Geometry check sheet. Reference: the model listing, model coordinates, mm. A direction names the side the tool comes from. Give positions to 0.01 mm unless a question says otherwise; leave off trailing zeros. Loops run counter-clockwise (first coordinate to the right, second up) from the corner with the lowest first, then second, coordinate; pieces in that order, holes last. Notation, with made-up numbers: (-33.5, 89) -> (23.5, 89) arc R29 cw to (23.5, 110) -> close; hole circle Ø2 at (4.25, -2). An arc over 180 degrees is marked (long way). One line per question, with ' | ' between items.
from build123d import *

# Parameters (mm, degrees)
SKETCH1_W                = 18
SKETCH1_H                = 40
BOSS_EXTRUDE1_DEPTH      = 6
BOSS_EXTRUDE2_DEPTH      = 14
SKETCH3_R                = 4.125
CUT_EXTRUDE1_DEPTH       = 30.681644159
FILLET1_R                = 7
SKETCH12_W               = 3
SKETCH12_H               = 8.5
CUT_EXTRUDE7_DEPTH       = 11.875
SKETCH13_R               = 1.5
CUT_EXTRUDE8_DEPTH       = 25.940241077
CUT_EXTRUDE9_REACH       = 32.725
SKETCH14_R               = 3
CUT_EXTRUDE10_REACH      = 35.526
SKETCH15_W               = 7
SKETCH15_H               = 5.5
SKETCH7_W                = 15.875
SKETCH7_H                = 6
BOSS_EXTRUDE3_DEPTH      = 7
FILLET2_R                = 7
SKETCH8_R                = 2.625
CUT_EXTRUDE4_DEPTH       = 30.189039039
BOSS_EXTRUDE4_DEPTH      = 2.5
BOSS_EXTRUDE4_DEPTH_BACK = 2.5
SKETCH10_R               = 4.875
CUT_EXTRUDE5_DEPTH       = 3


with BuildPart() as part:
    # Sketch1 → Boss-Extrude1 (new body)
    with BuildSketch(Plane(origin=(0, 0, 0), x_dir=(1, 0, 0), z_dir=(0, 1, 0))):
        Rectangle(SKETCH1_W, SKETCH1_H)
    extrude(amount=BOSS_EXTRUDE1_DEPTH)

    # Sketch2 → Boss-Extrude2 (add)
    with BuildSketch(Plane(origin=(0, 6, 0), x_dir=(1, 0, 0), z_dir=(0, 1, 0))):
        with BuildLine():
            Line((3, -20), (3, -8))
            ThreePointArc((3, -8), (-1, 0), (3, 8))
            Line((3, 8), (3, 20))
            Line((3, 20), (9, 20))
            Line((9, 20), (9, -20))
            Line((9, -20), (3, -20))
        make_face()
    extrude(amount=BOSS_EXTRUDE2_DEPTH)

    # Sketch3 → Cut-Extrude1 (cut, through all)
    with BuildSketch(Plane(origin=(0, 20, 0), x_dir=(1, 0, 0), z_dir=(0, 1, 0))):
        with Locations((9, 0)):
            Circle(SKETCH3_R)
    extrude(amount=-CUT_EXTRUDE1_DEPTH, mode=Mode.SUBTRACT)

    # Fillet1
    fillet1_edges = [part.edges().sort_by_distance(p)[0] for p in [
        (6, 20, 20),
        (6, 20, -20),
    ]]
    fillet(fillet1_edges, radius=FILLET1_R)

    # Sketch12 → Cut-Extrude7 (cut)
    with BuildSketch(Plane(origin=(0, 20, 0), x_dir=(1, 0, 0), z_dir=(0, 1, 0))):
        with Locations((5.25, 13)):
            Rectangle(SKETCH12_W, SKETCH12_H)
        with Locations((5.25, -13)):
            Rectangle(SKETCH12_W, SKETCH12_H)
    extrude(amount=-CUT_EXTRUDE7_DEPTH, mode=Mode.SUBTRACT)

    # Sketch13 → Cut-Extrude8 (cut, through all)
    with BuildSketch(Plane(origin=(0, 8.125, 0), x_dir=(1, 0, 0), z_dir=(0, 1, 0))):
        with Locations(Location((5.25, 13, 0), (0, 0, 270))):
            Circle(SKETCH13_R)
        with Locations((5.25, -13)):
            Circle(SKETCH13_R)
    extrude(amount=-CUT_EXTRUDE8_DEPTH, mode=Mode.SUBTRACT)

    # Sketch14 → Cut-Extrude9 (cut, up to next)
    with BuildSketch(Plane.ZY.offset(-3), mode=Mode.PRIVATE) as cut_extrude9_sk1:
        with Locations((-13, 13)):
            Circle(SKETCH14_R)
    cut_extrude9_tool1 = extrude(cut_extrude9_sk1.sketch, amount=-CUT_EXTRUDE9_REACH, mode=Mode.PRIVATE) & part.part
    # Sketch14 → Cut-Extrude9 (cut, up to next)
    with BuildSketch(Plane.ZY.offset(-3), mode=Mode.PRIVATE) as cut_extrude9_sk2:
        with Locations((13, 13)):
            Circle(SKETCH14_R)
    cut_extrude9_tool2 = extrude(cut_extrude9_sk2.sketch, amount=-CUT_EXTRUDE9_REACH, mode=Mode.PRIVATE) & part.part
    add(cut_extrude9_tool1.solids().sort_by_distance((3, 13, -13))[0], mode=Mode.SUBTRACT)
    add(cut_extrude9_tool2.solids().sort_by_distance((3, 13, 13))[0], mode=Mode.SUBTRACT)

    # Sketch15 → Cut-Extrude10 (cut, up to next)
    with BuildSketch(Plane(origin=(9, 0, 0), x_dir=(0, 0, -1), z_dir=(1, 0, 0)), mode=Mode.PRIVATE) as cut_extrude10_sk1:
        with Locations((13, 13)):
            Rectangle(SKETCH15_W, SKETCH15_H)
    cut_extrude10_tool1 = extrude(cut_extrude10_sk1.sketch, amount=-CUT_EXTRUDE10_REACH, mode=Mode.PRIVATE) & part.part
    # Sketch15 → Cut-Extrude10 (cut, up to next)
    with BuildSketch(Plane(origin=(9, 0, 0), x_dir=(0, 0, -1), z_dir=(1, 0, 0)), mode=Mode.PRIVATE) as cut_extrude10_sk2:
        with Locations((-13, 13)):
            Rectangle(SKETCH15_W, SKETCH15_H)
    cut_extrude10_tool2 = extrude(cut_extrude10_sk2.sketch, amount=-CUT_EXTRUDE10_REACH, mode=Mode.PRIVATE) & part.part
    add(cut_extrude10_tool1.solids().sort_by_distance((9, 13, -13))[0], mode=Mode.SUBTRACT)
    add(cut_extrude10_tool2.solids().sort_by_distance((9, 13, 13))[0], mode=Mode.SUBTRACT)

    # Sketch7 → Boss-Extrude3 (add)
    with BuildSketch(Plane(origin=(9, 0, 0), x_dir=(0, 0, -1), z_dir=(1, 0, 0))):
        with Locations((-12.0625, 3)):
            Rectangle(SKETCH7_W, SKETCH7_H)
        with Locations((12.0625, 3)):
            Rectangle(SKETCH7_W, SKETCH7_H)
    extrude(amount=BOSS_EXTRUDE3_DEPTH)

    # Fillet2
    fillet2_edges = [part.edges().sort_by_distance(p)[0] for p in [
        (-9, 3, -20),
        (16, 3, -20),
        (16, 3, 20),
        (-9, 3, 20),
        (16, 3, -4.125),
        (16, 3, 4.125),
    ]]
    fillet(fillet2_edges, radius=FILLET2_R - 0.0001)  # a hair under: the kernel refuses the full size

    # Sketch8 → Cut-Extrude4 (cut, through all)
    with BuildSketch(Plane(origin=(0, 6, 0), x_dir=(1, 0, 0), z_dir=(0, 1, 0))):
        with Locations(Location((-2, 13, 0), (0, 0, 270))):
            Circle(SKETCH8_R)
        with Locations(Location((-2, -13, 0), (0, 0, 90))):
            Circle(SKETCH8_R)
    extrude(amount=-CUT_EXTRUDE4_DEPTH, mode=Mode.SUBTRACT)

    # Sketch9 → Boss-Extrude4 (add, two sides: drawn at the far end of the back side and taken through both)
    with BuildSketch(Plane.XY.offset(-BOSS_EXTRUDE4_DEPTH_BACK)):
        Polygon((-9, 6), (2, 17), (2, 6), align=None)
    extrude(amount=BOSS_EXTRUDE4_DEPTH + BOSS_EXTRUDE4_DEPTH_BACK)

    # Sketch10 → Cut-Extrude5 (cut)
    with BuildSketch(Plane(origin=(0, 6, 0), x_dir=(1, 0, 0), z_dir=(0, 1, 0))):
        with Locations(Location((-2, 13, 0), (0, 0, 270))):
            Circle(SKETCH10_R)
        with Locations(Location((-2, -13, 0), (0, 0, 90))):
            Circle(SKETCH10_R)
    extrude(amount=-CUT_EXTRUDE5_DEPTH, mode=Mode.SUBTRACT)


solid = part.part
Item 1: Set-up check for faces 4 (the face through (8, 13, -16.5)), 5 (the face through (3.4, 11.2, -15.4)), 6 (the face through (2.834, 4.521, -13.635)), 7 (the face through (9, 10, -12)), 8 (the face through (-6, 6, -9)): record each of +Z, -Z, +X, -X, +Y, -Y from which the full face is reachable in a straight line by a thin tool's end or side.
Result:
face 4: +X | face 5: -X | face 6: +Y | face 7: +Z, -Z, +X, +Y | face 8: -Z, -X, +Y
Item 2: Release check for a two-part mould opening along Y. For faces 1 (the face through (-5, 10, 0)), 2 (the face through (14.004, 3.042, -6.23)), 3 (the face through (8, 13, -9.5)) record: pulls with the +Y half, pulls with the -Y half, needs draft (parallel to the pull), parting line crosses it, or undercut.
Result:
face 1: pulls with the +Y half | face 2: needs draft | face 3: undercut
Item 3: Depth check by flat-ended pin: pin 1 Ø7.5 at (x, z) = (12, -11) entering from +Y; pin 2 Ø2 at (x, z) = (14, 10) entering from +Y; pin 3 Ø3 at (x, z) = (-3, -1) entering from +Y; pin 4 Ø9.5 at (y, z) = (11, 12.5) entering from -X. Enter the tip coordinate at first touch or a pass-through.
Result:
pin 1: y = 20 | pin 2: y = 6 | pin 3: y = 13.5 | pin 4: x = 2.68
Item 4: Sectioned sample at B-B (z = 0). Record the cut outline in (x, y) (3 decimals), plus the area to 4 significant figures.
Result:
outline: (-9, 0) -> (4.875, 0) -> (4.875, 20) -> (-1, 20) -> (-1, 14) -> (-9, 6) -> close | area: 197.5 mm2
Item 5: Scan lines: probe 1 along Z at (x, y) = (4.5, 9.25); probe 2 along X at (y, z) = (1.9, 13) (3 decimals); probe 3 along X at (y, z) = (16.75, 16.5). Record each from-to range of solid material in increasing order.
Result:
probe 1: -20 to -17.25, -8.75 to 8.75, 17.25 to 20 | probe 2: -9 to -4.625, 0.625 to 3.75, 6.75 to 16 | probe 3: 3 to 3.75, 6.75 to 9
Item 6: Sectioned sample at A-A (x = -0.25). Record the cut outline in (y, z).
Result:
outline: (0, -20) -> (6, -20) -> (6, -17.55) -> (3, -17.55) -> (3, -14.96) -> (0, -14.96) -> close; (0, -11.04) -> (3, -11.04) -> (3, -8.45) -> (6, -8.45) -> (6, -3.8) -> (20, -3.8) -> (20, 3.8) -> (6, 3.8) -> (6, 8.45) -> (3, 8.45) -> (3, 11.04) -> (0, 11.04) -> close; (0, 14.96) -> (3, 14.96) -> (3, 17.55) -> (6, 17.55) -> (6, 20) -> (0, 20) -> close
